Answer from the drawing. Dimensions are ordinates in mm from the lowest x, y and z of the part. Give positions to 0.01 mm unless a question says otherwise; leave off trailing zeros. Order: outer loops, then holes, each group sorted by start corner. A loop starts at its lowest first (then second) coordinate and runs counter-clockwise, first axis right, second up. Notation, with made-up numbers: (-38.75, 43.5) - (12.25, 43.5) arc R6 cw to (12.25, 54.5) - close; hole circle Ø9 at (27, 57.5). An arc over 180 degrees is marked (long way). Answer in a Markdown table with one row per item.
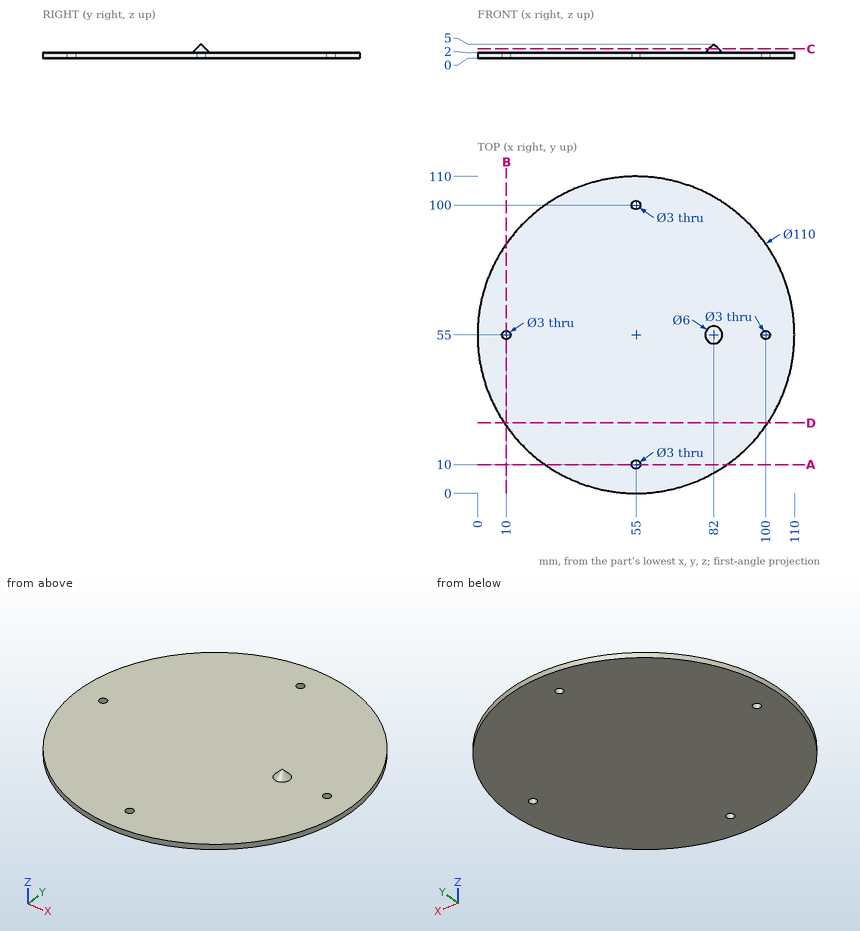
Item 1: Consider line 1 (Y direction, x = 55, z = 1.4); line 2 (Z direction, x = 91, y = 30.5); line 3 (X direction, y = 10, z = 0.55). Determine where each line is inside the solid, lowest interval first.
Answer block:
| item | result |
|---|---|
| line 1 | 0 to 8.5, 11.5 to 98.5, 101.5 to 110 |
| line 2 | 0 to 2 |
| line 3 | 23.38 to 53.5, 56.5 to 86.62 |
Item 2: Each of these flat-tipped pins is pushed along its axis until it touches: P1, Ø3, axis at y = 73, z = 1, coming from the +X side; P2, Ø2, axis at y = 73.5, z = 1.5, coming from the -X side; P3, Ø3.5, axis at x = 55, y = 100, coming from the +Z side. Where does it stop, or does it pass through?
Answer block:
| item | result |
|---|---|
| P1 | x = 107.47 |
| P2 | x = 2.86 |
| P3 | z = 2 |
Item 3: Find section C-C on z = 3.35. Write down the section's boundary in (x, y), then the cut area to 3 significant figures.
Answer block:
| item | result |
|---|---|
| outline | circle Ø3.3 at (82, 55) |
| area | 8.55 mm² |
Item 4: Find section A-A on y = 10. Write down the section's boundary in (x, z).
Answer block:
| item | result |
|---|---|
| outline | (23.38, 0) - (53.5, 0) - (53.5, 2) - (23.38, 2) - close; (56.5, 0) - (86.62, 0) - (86.62, 2) - (56.5, 2) - close |
Item 5: Find section D-D on y = 24.5. Write down the section's boundary in (x, z).
Answer block:
| item | result |
|---|---|
| outline | (9.23, 0) - (100.77, 0) - (100.77, 2) - (9.23, 2) - close |
